Build history of the part. All positions in model axes, mm. Give positions to 0.01 mm unless a question says otherwise; leave off trailing zeros. Write each loop counter-clockwise with the first axis right and the second up, starting at its lowest first coordinate (ties: lowest second). Pieces come first, ordered by that corner, then holes. Notation, with made-up numbers: M -16,83.5 L 43,83.5 A16 cw 43,99.5 Z; hole C -11,33 d10. An arc over 180 degrees is marked long. Return JSON: item names as keys, results as strings. Group by question number.
Q1. Band-saw the part on B-B, the plane y = 21. Count the separate pieces of the cut face and the enclosed holes in it, then the cut area to 3 significant figures.
Q2. Band-saw the part on A-A, the plane x = 13.5. Give the cut face in (y, z), then the cut area to 3 significant figures.
Q3. Wall check: probe 1 along X at (y, z) = (-21, 9.65); probe 2 along Y at (x, z) = (39, 10.25); probe 3 along Y at (x, z) = (-39, 10.25). Give the ranges that are in metal, low to high.
Q4. Flat gauge pins, fed straight in: pin 1 Ø2.5 at (x, y) = (-39, 21) entering from +Z; pin 2 Ø3.5 at (x, y) = (39, -21) entering from +Z. Where does each tip first touch, or does it go through?
Q5. Band-saw the part on C-C, the plane y = 0. Give the cut face in (x, z), then the cut area to 3 significant figures.
from build123d import *

# Parameters (mm, degrees)
PAD007_DEPTH    = 4
SKETCH018_R     = 1.6
SKETCH018_W     = 70
SKETCH018_H     = 51
SKETCH018_W_2   = 4
SKETCH018_H_2   = 6
POCKET005_DEPTH = 4
CHAMFER006_SIZE = 0.4
CHAMFER009_SIZE = 0.6


with BuildPart() as part:
    # Sketch017 → Pad007 (new body)
    with BuildSketch(Plane.XY):
        with BuildLine():
            Line((-40.5, -27), (40.5, -27))
            ThreePointArc((40.5, -27), (43.681981, -25.681981), (45, -22.5))
            Line((45, -22.5), (45, 22.5))
            ThreePointArc((45, 22.5), (43.681981, 25.681981), (40.5, 27))
            Line((40.5, 27), (-40.5, 27))
            ThreePointArc((-40.5, 27), (-43.681981, 25.681981), (-45, 22.5))
            Line((-45, 22.5), (-45, -22.5))
            ThreePointArc((-45, -22.5), (-43.681981, -25.681981), (-40.5, -27))
        make_face()
    extrude(amount=PAD007_DEPTH)

    # Sketch018 (on Face9 of Pad007) → Pocket005 (cut)
    with BuildSketch(Plane(origin=(0, 0, 0), x_dir=(1, 0, 0), z_dir=(0, 0, -1))):
        with Locations((-39, 21)):
            Circle(SKETCH018_R)
        with Locations((39, 21)):
            Circle(SKETCH018_R)
        with Locations((39, -21)):
            Circle(SKETCH018_R)
        with Locations((-39, -21)):
            Circle(SKETCH018_R)
        Rectangle(SKETCH018_W, SKETCH018_H)
        with Locations((-39, 14)):
            Rectangle(SKETCH018_W_2, SKETCH018_H_2)
    extrude(amount=-POCKET005_DEPTH, mode=Mode.SUBTRACT)

    # Chamfer006
    chamfer006_edges = [part.edges().sort_by_distance(p)[0] for p in [
        (0, -27, 0),
        (-43.681981, -25.681981, 0),
        (43.681981, -25.681981, 0),
        (-45, 0, 0),
        (45, 0, 0),
        (-43.681981, 25.681981, 0),
        (43.681981, 25.681981, 0),
        (0, 27, 0),
        (-40.6, -21, 0),
        (-41, -14, 0),
        (-39, -17, 0),
        (-37, -14, 0),
        (-39, -11, 0),
        (37.4, -21, 0),
        (-40.6, 21, 0),
        (-35, 0, 0),
        (0, -25.5, 0),
        (35, 0, 0),
        (0, 25.5, 0),
        (37.4, 21, 0),
        (-40.6, -21, 4),
        (-39, -17, 4),
        (-41, -14, 4),
        (-39, -11, 4),
        (-37, -14, 4),
        (-40.6, 21, 4),
        (37.4, 21, 4),
        (37.4, -21, 4),
    ]]
    chamfer(chamfer006_edges, length=CHAMFER006_SIZE)

    # Chamfer009
    chamfer009_edges = [part.edges().sort_by_distance(p)[0] for p in [
        (-45, 0, 4),
    ]]
    chamfer(chamfer009_edges, length=CHAMFER009_SIZE)


with BuildPart() as part_1:
    # Body001 placement: moved
    add(part.part.moved(Location((0, 0, 8.5))))


solid = part_1.part
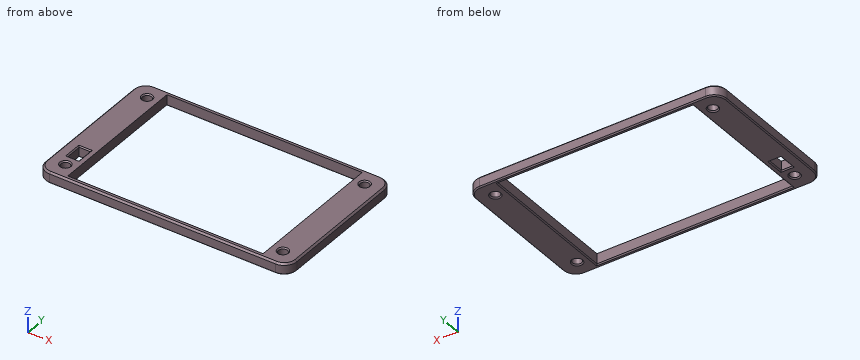
From the geometry:
{
 "1": {"separate pieces": "4", "enclosed holes": "0", "area": "53.1 mm^2"},
 "2": {"outline": "M -27,8.9 L -26.6,8.5 L -25.9,8.5 L -25.5,8.9 L -25.5,12.5 L -26.4,12.5 L -27,11.9 Z; M 25.5,8.9 L 25.9,8.5 L 26.6,8.5 L 27,8.9 L 27,11.9 L 26.4,12.5 L 25.5,12.5 Z", "area": "11.3 mm^2"},
 "3": {"probe 1": "x = -45 to -40.6, -37.4 to -35, 35 to 37.4, 40.6 to 45", "probe 2": "y = -27 to -22.6, -19.4 to 19.4, 22.6 to 27", "probe 3": "y = -27 to -22.6, -19.4 to -17, -11 to 19.4, 22.6 to 27"},
 "4": {"pin 1": "passes through", "pin 2": "stops at z = 12.25"},
 "5": {"outline": "M -45,8.9 L -44.6,8.5 L -35.4,8.5 L -35,8.9 L -35,12.5 L -44.4,12.5 L -45,11.9 Z; M 35,8.9 L 35.4,8.5 L 44.6,8.5 L 45,8.9 L 45,11.9 L 44.4,12.5 L 35,12.5 Z", "area": "79.3 mm^2"}
}
